Check sheet for the modelled part. Datum: model origin and axes. Units: mm. Coordinates: 2 decimals unless noted, no trailing zeros. Order: outer loops, then holes, each group sorted by start corner. A loop starts at its lowest first (then second) coordinate and runs counter-clockwise, first axis right, second up.
from build123d import *

# Parameters (mm, degrees)
SKETCH1_R               = 25
SKETCH1_R_2             = 21
BOSS_EXTRUDE1_DEPTH     = 145
CHAMFER1_SIZE           = 3
SKETCH2_R               = 11
CUT_EXTRUDE1_DEPTH      = 26
CUT_EXTRUDE1_DEPTH_BACK = 26
SKETCH3_R               = 6
CUT_EXTRUDE2_DEPTH      = 26.0000001
CUT_EXTRUDE2_DEPTH_BACK = 26.0000001
CUT_EXTRUDE3_REACH      = 27
SKETCH4_W               = 6
SKETCH4_H               = 75


with BuildPart() as part:
    # Sketch1 → Boss-Extrude1 (new body, symmetric)
    with BuildSketch(Plane.XY):
        Circle(SKETCH1_R)
        Circle(SKETCH1_R_2, mode=Mode.SUBTRACT)
    extrude(amount=BOSS_EXTRUDE1_DEPTH, both=True)

    # Chamfer1
    chamfer1_edges = [part.edges().sort_by_distance(p)[0] for p in [
        (-25, 0, 145),
    ]]
    chamfer(chamfer1_edges, length=CHAMFER1_SIZE)

    # Sketch2 → Cut-Extrude1 (cut, two sides)
    with BuildSketch(Plane(origin=(0, 0, 0), x_dir=(1, 0, 0), z_dir=(0, 1, 0))) as cut_extrude1_sk:
        with Locations((0, 110)):
            Circle(SKETCH2_R)
    extrude(amount=CUT_EXTRUDE1_DEPTH, mode=Mode.SUBTRACT)
    extrude(cut_extrude1_sk.sketch, amount=-CUT_EXTRUDE1_DEPTH_BACK, mode=Mode.SUBTRACT)

    # Sketch3 → Cut-Extrude2 (cut, two sides)
    with BuildSketch(Plane(origin=(0, 0, 0), x_dir=(0, 0, -1), z_dir=(1, 0, 0))) as cut_extrude2_sk:
        with Locations((125, 0)):
            Circle(SKETCH3_R)
    extrude(amount=CUT_EXTRUDE2_DEPTH, mode=Mode.SUBTRACT)
    extrude(cut_extrude2_sk.sketch, amount=-CUT_EXTRUDE2_DEPTH_BACK, mode=Mode.SUBTRACT)

    # Sketch4 → Cut-Extrude3 (cut, up to next)
    with BuildSketch(Plane(origin=(0, 0, 0), x_dir=(1, 0, 0), z_dir=(0, 1, 0)), mode=Mode.PRIVATE) as cut_extrude3_sk1:
        with Locations((0, -57.5)):
            Rectangle(SKETCH4_W, SKETCH4_H)
    cut_extrude3_tool1 = extrude(cut_extrude3_sk1.sketch, amount=-CUT_EXTRUDE3_REACH, mode=Mode.PRIVATE) & part.part
    add(cut_extrude3_tool1.solids().sort_by_distance((0, 0, 57.5))[0], mode=Mode.SUBTRACT)


solid = part.part
(1) Cross-section at B-B (y = 0). Enter the section's corners in (x, z), and give its area (4 significant figures).
Filled in:
outline: (-25, -145) - (-21, -145) - (-21, -131) - (-25, -131) - close; (-25, -119) - (-21, -119) - (-21, 145) - (-22, 145) - (-25, 142) - close; (21, -145) - (25, -145) - (25, -131) - (21, -131) - close; (21, -119) - (25, -119) - (25, 142) - (22, 145) - (21, 145) - close
area: 2,215 mm2
(2) Cross-section at C-C (z = -125). Enter the section's corners in (x, y), and give its area (3 significant figures).
Filled in:
outline: (-24.27, -6) arc R25 ccw to (24.27, -6) - (20.12, -6) arc R21 cw to (-20.12, -6) - close; (-24.27, 6) - (-20.12, 6) arc R21 cw to (20.12, 6) - (24.27, 6) arc R25 ccw to start
area: 481 mm2
(3) Cross-section at D-D (z = -34). Enter the section's corners in (x, y).
Filled in:
outline: circle Ø50 at (0, 0); hole circle Ø42 at (0, 0)
(4) Go/stop test with flat-tipped pins: P1, Ø10, axis at y = -5.5, z = -68.5, coming from the +X side (3 decimals); P2, Ø3, axis at x = -19, z = 33, coming from the +Y side; P3, Ø2, axis at x = 7, z = 61.5, coming from the -Y side. Record where each tip stops, or that it passes through.
Filled in:
P1: stops at x = 24.995
P2: stops at y = 17.85
P3: stops at y = -24.27
(5) Thickness scan on probe 1 along Z at (x, y) = (21.85, 0); probe 2 along X at (y, z) = (0, 32.5); probe 3 along X at (y, z) = (1.5, 28). Record the ranges inside material, lowest first.
Filled in:
probe 1: z = -145 to -131, -119 to 145
probe 2: x = -25 to -21, 21 to 25
probe 3: x = -24.95 to -20.95, 20.95 to 24.95
(6) Cross-section at A-A (x = 0). Enter the section's corners in (y, z), and give its area (4 significant figures).
Filled in:
outline: (-25, -145) - (-21, -145) - (-21, -121) - (-25, -121) - close; (-25, -99) - (-21, -99) - (-21, 20) - (-25, 20) - close; (-25, 95) - (-21, 95) - (-21, 145) - (-22, 145) - (-25, 142) - close; (21, -145) - (25, -145) - (25, -121) - (21, -121) - close; (21, -99) - (25, -99) - (25, 142) - (22, 145) - (21, 145) - close
area: 1,835 mm2
(7) Release check for a two-part mould opening along X. For faces 1 (the flat face through (-5.7, 20.5, -145)), 2 (the cylindrical face through (-1.432, -21.404, -120.906)), 3 (the cylindrical face through (23.846, 7.509, 0.509)) record: +X half, -X half, draft (parallel to the pull), parting line (faces both ways), or undercut.
Filled in:
face 1: draft
face 2: undercut
face 3: parting line
